```python
from build123d import *

# Parameters (mm, degrees)
ESQUISSE1_W                  = 113.5
ESQUISSE1_H                  = 25
BOSS_EXTRU_1_DEPTH           = 15
BOSS_EXTRU_2_DEPTH           = 9.5
BOSS_EXTRU_2_DEPTH_BACK      = 9.5
BOSS_EXTRU_3_DEPTH           = 13
ENL_V_MAT_EXTRU_1_DEPTH      = 125.142055726
ENL_V_MAT_EXTRU_1_DEPTH_BACK = 125.142055726
ESQUISSE2_W                  = 6.5
ESQUISSE2_H                  = 11.5
CONG_1_R                     = 2.5


with BuildPart() as part:
    # Esquisse1 → Boss.-Extru.1 (new, symmetric)
    with BuildSketch(Plane(origin=(0, 0, 0), x_dir=(1, 0, 0), z_dir=(0, 1, 0))):
        with Locations((-56.75, 0)):
            Rectangle(ESQUISSE1_W, ESQUISSE1_H)
    extrude(amount=BOSS_EXTRU_1_DEPTH, both=True)

    # Esquisse1<3> → Boss.-Extru.2 (add, two sides: drawn at the far end of the back side and taken through both)
    # profile 1 of 2: a face of its own
    with BuildSketch(Plane(origin=(0, 0, 0), x_dir=(1, 0, 0), z_dir=(0, 1, 0)).offset(-BOSS_EXTRU_2_DEPTH_BACK)):
        Polygon((12.644707776, -12.5), (0, -12.5), (-113.5, -12.5), (-113.5, -48), (-4.5, -48), (-4.5, -31), (25.598547233, -31), align=None)
        with BuildLine():
            Line((-31, -36), (-83, -36))
            ThreePointArc((-83, -36), (-88.5, -30.5), (-83, -25))
            Line((-83, -25), (-31, -25))
            ThreePointArc((-31, -25), (-25.5, -30.5), (-31, -36))
        make_face(mode=Mode.SUBTRACT)
    # profile 2 of 2: a face of its own
    with BuildSketch(Plane(origin=(0, 0, 0), x_dir=(1, 0, 0), z_dir=(0, 1, 0)).offset(-BOSS_EXTRU_2_DEPTH_BACK)):
        Polygon((-113.5, 12.5), (0, 12.5), (12.644707776, 12.5), (25.598547233, 31), (-4.5, 31), (-4.5, 48), (-113.5, 48), align=None)
        with BuildLine():
            ThreePointArc((-83, 25), (-88.5, 30.5), (-83, 36))
            Line((-83, 36), (-31, 36))
            ThreePointArc((-31, 36), (-25.5, 30.5), (-31, 25))
            Line((-31, 25), (-83, 25))
        make_face(mode=Mode.SUBTRACT)
    extrude(amount=BOSS_EXTRU_2_DEPTH + BOSS_EXTRU_2_DEPTH_BACK)

    # Esquisse1<4> → Boss.-Extru.3 (add, symmetric)
    with BuildSketch(Plane(origin=(0, 0, 0), x_dir=(1, 0, 0), z_dir=(0, 1, 0))):
        Polygon((-4.5, 31), (25.598547233, 31), (30.5, 38), (30.5, 48), (-4.5, 48), align=None)
        Polygon((30.5, -38), (25.598547233, -31), (-4.5, -31), (-4.5, -48), (30.5, -48), align=None)
    extrude(amount=BOSS_EXTRU_3_DEPTH, both=True)

    # Esquisse2 → Enlèv. mat.-Extru.1 (cut, two sides: drawn at the far end of the back side and taken through both)
    with BuildSketch(Plane.XY.offset(-ENL_V_MAT_EXTRU_1_DEPTH_BACK)):
        with Locations((-110.25, -9.25)):
            Rectangle(ESQUISSE2_W, ESQUISSE2_H)
    extrude(amount=ENL_V_MAT_EXTRU_1_DEPTH + ENL_V_MAT_EXTRU_1_DEPTH_BACK, mode=Mode.SUBTRACT)

    # Congé1
    cong_1_edges = [part.edges().sort_by_distance(p)[0] for p in [
        (-57, 9.5, 36),
        (-57, -9.5, 36),
        (-88.5, 9.5, 30.5),
        (-57, 9.5, 25),
        (-25.5, 9.5, 30.5),
        (-57, -9.5, 25),
        (-88.5, -9.5, 30.5),
        (-25.5, -9.5, 30.5),
        (-25.5, 9.5, -30.5),
        (-25.5, -9.5, -30.5),
        (-57, 9.5, -25),
        (-57, -9.5, -25),
        (-88.5, 9.5, -30.5),
        (-88.5, -9.5, -30.5),
        (-57, 9.5, -36),
        (-57, -9.5, -36),
    ]]
    fillet(cong_1_edges, radius=CONG_1_R)


solid = part.part
```
Work out the finished part from the listing and answer in its coordinate system (mm). A direction names the side the tool comes from. Give positions to 0.01 mm unless a question says otherwise; leave off trailing zeros. Order: outer loops, then holes, each group sorted by start corner. A loop starts at its lowest first (then second) coordinate and runs counter-clockwise, first axis right, second up. Notation, with made-up numbers: M -17,41 L -8,41 A17 cw -8,49 Z; hole C 56.5,44.5 d3. An arc over 180 degrees is marked long. Return JSON: item names as keys, results as strings.
1) Section B-B, the plane z = 6.5 is taken. Write down the section's boundary in (x, y).
Resolved:
{"outline": "M -113.5,-3.5 L -107,-3.5 L -107,-15 L 0,-15 L 0,15 L -113.5,15 Z"}
2) Straight lines are drawn through the part: line 1 along Z through (x, y) = (-75, -6.75); line 2 along Z through (x, y) = (-79, -8); line 3 along Z through (x, y) = (16, -12.25). For each, find the intervals that lie inside material, in ascending order. Write a range as [from, to].
Resolved:
{"line 1": "[-48, -36], [-25, 25], [36, 48]", "line 2": "[-48, -36.21], [-24.79, 24.79], [36.21, 48]", "line 3": "[-48, -31], [31, 48]"}
3) Section A-A, the plane y = 4 is taken. Write down the section's boundary in (x, z).
Resolved:
{"outline": "M -113.5,-48 L 30.5,-48 L 30.5,-38 L 12.64,-12.5 L 0,-12.5 L 0,12.5 L 12.64,12.5 L 30.5,38 L 30.5,48 L -113.5,48 Z; hole M -83,-36 L -31,-36 A5.5 ccw -31,-25 L -83,-25 A5.5 ccw Z; hole M -83,25 L -31,25 A5.5 ccw -31,36 L -83,36 A5.5 ccw Z"}
4) Each of these flat-tipped pins is pushed along its axis until it touches: pin 1 (10 mm diameter, centred on y = 1.5, z = -13.5, fed in from +X); pin 2 (4.5 mm diameter, centred on x = -59, y = 11, fed in from -Z); pin 3 (1.8 mm diameter, centred on y = -11.5, z = 36.5, fed in from -X); pin 4 (1.6 mm diameter, centred on x = -35, y = -12.5, fed in from +Z). Where does it stop, or does it pass through?
Resolved:
{"pin 1": "x = 16.85", "pin 2": "z = -48", "pin 3": "x = -4.5", "pin 4": "z = 12.5"}
5) For a pull along Z with two mould halves and no side action, classify faces 1 (the cylindrical face through (-25.5, -0.1, -30.6)), 2 (the flat face through (30.5, 0, -43)), 3 (the flat face through (-43, 0, 48)) as +Z half, -Z half, draft (parallel to the pull), parting line (faces both ways), or undercut.
Resolved:
{"face 1": "undercut", "face 2": "draft", "face 3": "+Z half"}
6) A tool of negligible diameter and unlimited length cuts with its end or side. For faces 4 (the flat face through (-4.5, -11, -40)), 5 (the flat face through (-4.5, 11, 39)), 6 (the flat face through (-4.5, -11, 39)), 7 (the flat face through (-57, 0, -25)), 8 (the flat face through (0, 0, 0)), from which of +Z, -Z, +X, -X, +Y, -Y can it reach the whole face along a straight path? Write none if from no direction.
Resolved:
{"face 4": "-Z, -X, -Y", "face 5": "+Z, -X, +Y", "face 6": "+Z, -X, -Y", "face 7": "+Y, -Y", "face 8": "+X, +Y, -Y"}
